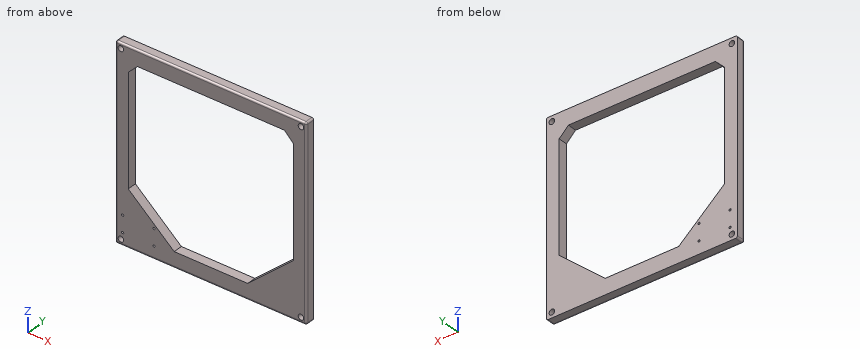
```python
from build123d import *

# Parameters (mm, degrees)
F0_W      = 104
F0_H      = 104
F0_R      = 1.5
F2_DEPTH  = 5
F2_FACE_W = 104
F2_FACE_H = 104
F2_FACE_R = 1.5
F3_DEPTH  = 25
F4_R      = 1
F5_R      = 0.6
F6_DEPTH  = 25


with BuildPart() as f2:
    # F0 (on Front) → F2 (new body)
    with BuildSketch(Plane.XZ):
        Rectangle(F0_W, F0_H)
        with Locations((-49, -49)):
            Circle(F0_R, mode=Mode.SUBTRACT)
        with Locations((49, -49)):
            Circle(F0_R, mode=Mode.SUBTRACT)
        with Locations((-49, 49)):
            Circle(F0_R, mode=Mode.SUBTRACT)
        with Locations((49, 49)):
            Circle(F0_R, mode=Mode.SUBTRACT)
    extrude(amount=F2_DEPTH)

    # F1 (on Front) + F2_face (on face) → F3 (cut)
    with BuildSketch(Plane.XZ):
        Polygon((40, 43.5), (-40, 43.5), (-45, 38.5), (-45, -21.5), (-20, -43.5), (20, -43.5), (45, -21.5), (45, 38.5), align=None)
    with BuildSketch(Plane.XZ.offset(5)):
        Rectangle(F2_FACE_W, F2_FACE_H)
        with Locations((-49, -49)):
            Circle(F2_FACE_R, mode=Mode.SUBTRACT)
        with Locations((49, -49)):
            Circle(F2_FACE_R, mode=Mode.SUBTRACT)
        with Locations((-49, 49)):
            Circle(F2_FACE_R, mode=Mode.SUBTRACT)
        with Locations((49, 49)):
            Circle(F2_FACE_R, mode=Mode.SUBTRACT)
    extrude(amount=F3_DEPTH, mode=Mode.SUBTRACT)

    # F4
    f4_edges = [f2.edges().sort_by_distance(p)[0] for p in [
        (-52, -2.5, 52),
        (-52, -5, 0),
        (0, -5, 52),
        (-52, -2.5, -52),
        (0, -5, -52),
        (52, -5, 0),
        (52, -2.5, 52),
        (52, -2.5, -52),
    ]]
    fillet(f4_edges, radius=F4_R)

    # F5 (on face) → F6 (cut)
    with BuildSketch(Plane.XZ.offset(5)):
        with Locations((-48.035103, -36.183678)):
            Circle(F5_R)
        with Locations((-48.035103, -45.183678)):
            Circle(F5_R)
        with Locations((-31.035103, -36.183678)):
            Circle(F5_R)
        with Locations((-31.035103, -45.183678)):
            Circle(F5_R)
    extrude(amount=-F6_DEPTH, mode=Mode.SUBTRACT)


solid = f2.part
```
Input: part model. Units: mm. Frame: model coordinates. Give positions to 0.01 mm unless a question says otherwise; leave off trailing zeros. Order: outer loops, then holes, each group sorted by start corner. A loop starts at its lowest first (then second) coordinate and runs counter-clockwise, first axis right, second up. Notation, with made-up numbers: M 35.25,73 L 85.25,73 A21 cw 85.25,80 Z; hole C -7,85.25 d8. An arc over 180 degrees is marked long. Return JSON: item names as keys, results as strings.
Item 1: Cut plane C-C (z = 5). Return loops of the section in (x, y), then the cut area to 3 significant figures.
Solutions:
{"outline": "M -52,-4 A1 ccw -51,-5 L -45,-5 L -45,0 L -52,0 Z; M 45,-5 L 51,-5 A1 ccw 52,-4 L 52,0 L 45,0 Z", "area": "69.6 mm^2"}
Item 2: First-contact query: P1, Ø2.5, axis at x = 49, z = -49, coming from the -Y side. Flat tip, straight axial feed; report the tip coordinate or a pass-through.
Solutions:
{"P1": "through"}
Item 3: Cut plane B-B (z = -49). Return loops of the section in (x, y), then the cut area to 3 significant figures.
Solutions:
{"outline": "M -52,-4 A1 ccw -51,-5 L -50.5,-5 L -50.5,0 L -52,0 Z; M -47.5,-5 L 47.5,-5 L 47.5,0 L -47.5,0 Z; M 50.5,-5 L 51,-5 A1 ccw 52,-4 L 52,0 L 50.5,0 Z", "area": "490 mm^2"}
Item 4: Ray query, probe 1 along Z at (x, y) = (-49, -2); probe 2 along X at (y, z) = (-4.1, 8); probe 3 along Z at (x, y) = (-16, -1.55). Return the intervals inside material, ascending.
Solutions:
{"probe 1": "-52 to -50.5, -47.5 to 47.5, 50.5 to 52", "probe 2": "-51.99 to -45, 45 to 51.99", "probe 3": "-52 to -43.5, 43.5 to 52"}
Item 5: Cut plane A-A (x = -22.5). Return loops of the section in (y, z).
Solutions:
{"outline": "M -5,-51 A1 ccw -4,-52 L 0,-52 L 0,-41.3 L -5,-41.3 Z; M -5,43.5 L 0,43.5 L 0,52 L -4,52 A1 ccw -5,51 Z"}
Item 6: Cut plane D-D (x = 49). Return loops of the section in (y, z), then the cut area to 3 significant figures.
Solutions:
{"outline": "M -5,-51 A1 ccw -4,-52 L 0,-52 L 0,-50.5 L -5,-50.5 Z; M -5,-47.5 L 0,-47.5 L 0,47.5 L -5,47.5 Z; M -5,50.5 L 0,50.5 L 0,52 L -4,52 A1 ccw -5,51 Z", "area": "490 mm^2"}
